from build123d import *

# Parameters (mm, degrees)
SKETCH1_W               = 127
SKETCH1_H               = 63.5
BOSS_EXTRUDE1_DEPTH     = 1.5875
CUT_EXTRUDE2_DEPTH      = 72.066117982
CUT_EXTRUDE2_DEPTH_BACK = 72.066117982
SKETCH3_R               = 14.2875
CUT_EXTRUDE3_DEPTH      = 72.012904857
CUT_EXTRUDE3_DEPTH_BACK = 72.012904857
SKETCH4_R               = 2.54
CUT_EXTRUDE4_DEPTH      = 72.012904857
CUT_EXTRUDE4_DEPTH_BACK = 72.012904857
SKETCH5_R               = 2.54


with BuildPart() as part:
    # Sketch1 → Boss-Extrude1 (new, symmetric)
    with BuildSketch(Plane.XY):
        Rectangle(SKETCH1_W, SKETCH1_H)
    extrude(amount=BOSS_EXTRUDE1_DEPTH, both=True)

    # Sketch3 → Cut-Extrude2 (cut, two sides: drawn at the far end of the back side and taken through both)
    with BuildSketch(Plane.XY.offset(1.5875).offset(-CUT_EXTRUDE2_DEPTH_BACK)):
        with Locations((0, -10.125)):
            Circle(SKETCH3_R)
    extrude(amount=CUT_EXTRUDE2_DEPTH + CUT_EXTRUDE2_DEPTH_BACK, mode=Mode.SUBTRACT)

    # Sketch4 → Cut-Extrude3 (cut, two sides: drawn at the far end of the back side and taken through both)
    with BuildSketch(Plane.XY.offset(-CUT_EXTRUDE3_DEPTH_BACK)):
        with Locations((-50.8, 19.05)):
            Circle(SKETCH4_R)
        with Locations((-50.8, -19.05)):
            Circle(SKETCH4_R)
        with Locations((50.8, -19.05)):
            Circle(SKETCH4_R)
        with Locations((50.8, 19.05)):
            Circle(SKETCH4_R)
    extrude(amount=CUT_EXTRUDE3_DEPTH + CUT_EXTRUDE3_DEPTH_BACK, mode=Mode.SUBTRACT)

    # Sketch5 → Cut-Extrude4 (cut, two sides: drawn at the far end of the back side and taken through both)
    with BuildSketch(Plane.XY.offset(-CUT_EXTRUDE4_DEPTH_BACK)):
        with Locations((31.75, 19.05)):
            Circle(SKETCH5_R)
        with Locations((-31.75, 19.05)):
            Circle(SKETCH5_R)
        with Locations((-31.75, -19.05)):
            Circle(SKETCH5_R)
        with Locations((31.75, -19.05)):
            Circle(SKETCH5_R)
    extrude(amount=CUT_EXTRUDE4_DEPTH + CUT_EXTRUDE4_DEPTH_BACK, mode=Mode.SUBTRACT)


solid = part.part
Input: part model. Units: mm. Frame: model coordinates. Round coordinates to 2 decimals unless told otherwise and drop trailing zeros. Write each loop counter-clockwise with the first axis right and the second up, starting at its lowest first coordinate (ties: lowest second). Pieces come first, ordered by that corner, then holes.
1) Ray query, L1, parallel to Y at x = -31.75, z = -0.1; L2, parallel to X at y = -20.5, z = -1; L3, parallel to X at y = -19.05, z = -0.5. Return the intervals inside material, ascending.
2) Cut plane C-C (y = -12). Return the cut outline in (x, z), then the cut area to 3 significant figures.
3) Cut plane A-A (x = -50.8). Return the cut outline in (y, z).
4) Cut plane B-B (y = 19.05). Return the cut outline in (x, z).
5) Draft query along X for faces 1 (the cylindrical face through (31.2, 16.57, -0.02)), 2 (the flat face through (63.5, 0, 0)), 3 (the cylindrical face through (-33.62, -17.33, -0.02)), 4 (the flat face through (-1, 31.75, 0)). Return one class per face: pulls with the +X half, pulls with the -X half, needs draft (parallel to the pull), parting line crosses it, or undercut.
6) Cut plane D-D (x = 4). Return the cut outline in (y, z), then the cut area to 3 significant figures.
Geometry says:
1. L1: y = -31.75 to -21.59, -16.51 to 16.51, 21.59 to 31.75
1. L2: x = -63.5 to -52.89, -48.71 to -33.84, -29.66 to -9.82, 9.82 to 29.66, 33.84 to 48.71, 52.89 to 63.5
1. L3: x = -63.5 to -53.34, -48.26 to -34.29, -29.21 to -11.16, 11.16 to 29.21, 34.29 to 48.26, 53.34 to 63.5
2. outline: (-63.5, -1.59) - (-14.16, -1.59) - (-14.16, 1.59) - (-63.5, 1.59) - close; (14.16, -1.59) - (63.5, -1.59) - (63.5, 1.59) - (14.16, 1.59) - close
2. area: 313 mm2
3. outline: (-31.75, -1.59) - (-21.59, -1.59) - (-21.59, 1.59) - (-31.75, 1.59) - close; (-16.51, -1.59) - (16.51, -1.59) - (16.51, 1.59) - (-16.51, 1.59) - close; (21.59, -1.59) - (31.75, -1.59) - (31.75, 1.59) - (21.59, 1.59) - close
4. outline: (-63.5, -1.59) - (-53.34, -1.59) - (-53.34, 1.59) - (-63.5, 1.59) - close; (-48.26, -1.59) - (-34.29, -1.59) - (-34.29, 1.59) - (-48.26, 1.59) - close; (-29.21, -1.59) - (29.21, -1.59) - (29.21, 1.59) - (-29.21, 1.59) - close; (34.29, -1.59) - (48.26, -1.59) - (48.26, 1.59) - (34.29, 1.59) - close; (53.34, -1.59) - (63.5, -1.59) - (63.5, 1.59) - (53.34, 1.59) - close
5. face 1: undercut
5. face 2: pulls with the +X half
5. face 3: undercut
5. face 4: needs draft
6. outline: (-31.75, -1.59) - (-23.84, -1.59) - (-23.84, 1.59) - (-31.75, 1.59) - close; (3.59, -1.59) - (31.75, -1.59) - (31.75, 1.59) - (3.59, 1.59) - close
6. area: 115 mm2
